Source: CAD feature listing. Evaluate the final solid. Frame: model axes, mm. A direction names the side the tool comes from. Give positions to 0.01 mm unless a question says otherwise; leave off trailing zeros. Write each loop counter-clockwise with the first axis right and the second up, starting at its lowest first coordinate (ties: lowest second). Pieces come first, ordered by that corner, then holes. Notation, with made-up numbers: M -15,80 L -5,80 A10 ccw -5,86 Z; hole C 82.25,12.25 d1. An arc over 180 degrees is marked long. Return JSON: item names as keys, results as strings.
```python
from build123d import *

# Parameters (mm, degrees)
SKETCH2_W               = 200
SKETCH2_H               = 200
BOSS_EXTRUDE1_DEPTH     = 50
CUT_EXTRUDE1_DEPTH      = 151
CUT_EXTRUDE1_DEPTH_BACK = 15
SKETCH5_R               = 75.5
CUT_EXTRUDE2_DEPTH      = 146.688022843
CUT_EXTRUDE2_DEPTH_BACK = 146.688022843
SKETCH7_R               = 50.25
SKETCH12_R              = 20.123320675
BOSS_EXTRUDE2_DEPTH     = 50
CIRPATTERN1_COUNT       = 4
CIRPATTERN1_ANGLE       = 276
SKETCH13_R              = 1.5
CUT_EXTRUDE3_DEPTH      = 10
CIRPATTERN2_COUNT       = 6
BOSS_EXTRUDE3_START     = -8
SKETCH14_R              = 50.25
BOSS_EXTRUDE3_DEPTH     = 8


with BuildPart() as part:
    # Sketch2 → Boss-Extrude1 (new body)
    with BuildSketch(Plane(origin=(0, 0, 0), x_dir=(1, 0, 0), z_dir=(0, 1, 0))):
        Rectangle(SKETCH2_W, SKETCH2_H)
    extrude(amount=BOSS_EXTRUDE1_DEPTH)

    # Sketch5 → Cut-Extrude1 (cut, two sides: drawn at the far end of the back side and taken through both)
    with BuildSketch(Plane(origin=(0, 50, 0), x_dir=(1, 0, 0), z_dir=(0, 1, 0)).offset(-CUT_EXTRUDE1_DEPTH_BACK)):
        with Locations(Location((0, 0, 0), (0, 0, 90))):
            Circle(SKETCH5_R)
    extrude(amount=CUT_EXTRUDE1_DEPTH + CUT_EXTRUDE1_DEPTH_BACK, mode=Mode.SUBTRACT)

    # Sketch7 → Cut-Extrude2 (cut, two sides: drawn at the far end of the back side and taken through both)
    with BuildSketch(Plane(origin=(0, 35, 0), x_dir=(1, 0, 0), z_dir=(0, 1, 0)).offset(-CUT_EXTRUDE2_DEPTH_BACK)):
        with Locations(Location((0, 0, 0), (0, 0, 270))):
            Circle(SKETCH7_R)
    extrude(amount=CUT_EXTRUDE2_DEPTH + CUT_EXTRUDE2_DEPTH_BACK, mode=Mode.SUBTRACT)

    # Sketch12 → Boss-Extrude2 (add)
    with BuildSketch(Plane.XZ):
        with Locations(Location((-74.168810486, 63.963412144, 0), (0, 0, 270))):
            Circle(SKETCH12_R)
    boss_extrude2 = extrude(amount=BOSS_EXTRUDE2_DEPTH)

    # CirPattern1: Boss-Extrude2 ×4 about axis
    cirpattern1_axis = Axis((0, 0, 0), (0, 1, 0))
    for i in range(1, CIRPATTERN1_COUNT):
        add(boss_extrude2.rotate(cirpattern1_axis, i * CIRPATTERN1_ANGLE / (CIRPATTERN1_COUNT - 1)))

    # Sketch13 → Cut-Extrude3 (cut)
    with BuildSketch(Plane(origin=(0, 35, 0), x_dir=(1, 0, 0), z_dir=(0, 1, 0))):
        with Locations(Location((0, 65, 0), (0, 0, 270))):
            Circle(SKETCH13_R)
    cut_extrude3 = extrude(amount=-CUT_EXTRUDE3_DEPTH, mode=Mode.SUBTRACT)

    # CirPattern2: Cut-Extrude3 ×6 about axis
    cirpattern2_axis = Axis((0, 0, 0), (0, 1, 0))
    for i in range(1, CIRPATTERN2_COUNT):
        add(cut_extrude3.rotate(cirpattern2_axis, i * 360 / CIRPATTERN2_COUNT), mode=Mode.SUBTRACT)

    # Sketch14 → Boss-Extrude3 (add)
    with BuildSketch(Plane.XZ.offset(BOSS_EXTRUDE3_START)):
        with Locations(Location((0, 0, 0), (0, 0, 90))):
            Circle(SKETCH14_R)
    extrude(amount=BOSS_EXTRUDE3_DEPTH)


solid = part.part
```
1) Cut plane B-B, the plane y = 11.5. Return the cut outline in (x, z), then the cut area to 3 significant figures.
Numbers:
{"outline": "M -100,-100 L 100,-100 L 100,100 L -100,100 Z; hole C 0,0 d100.5", "area": "32,100 mm²"}
2) Cut plane D-D, the plane y = -33.5. Return the cut outline in (x, z).
Numbers:
{"outline": "C -74.17,63.96 d40.25; C -71.37,-67.08 d40.25; C 66.51,71.89 d40.25; C 69.53,-68.98 d40.25"}
3) Draft query along X for faces 1 (the face through (100, 25, 1)), 2 (the face through (-1, 0, -1)), 3 (the face through (49, 35, -16)), 4 (the face through (-74, -50, 64)). Return one class per face: released by +X, released by -X, zero draft, split by the parting line, or undercut.
Numbers:
{"face 1": "released by +X", "face 2": "undercut", "face 3": "undercut", "face 4": "zero draft"}
4) Cut plane A-A, the plane z = 0. Return the cut outline in (x, y), then the cut area to 3 significant figures.
Numbers:
{"outline": "M -100,0 L 100,0 L 100,50 L 75.5,50 L 75.5,35 L 50.25,35 L 50.25,8 L -50.25,8 L -50.25,35 L -75.5,35 L -75.5,50 L -100,50 Z", "area": "5,020 mm²"}
5) Cut plane C-C, the plane x = -14. Return the cut outline in (y, z), then the cut area to 3 significant figures.
Numbers:
{"outline": "M 0,-100 L 50,-100 L 50,-74.19 L 35,-74.19 L 35,-48.26 L 8,-48.26 L 8,48.26 L 35,48.26 L 35,74.19 L 50,74.19 L 50,100 L 0,100 Z", "area": "5,170 mm²"}
6) Contact query for flat-ended pins moving along their axis: pin 1 Ø8 at (x, z) = (68, 30.5) entering from +Y; pin 2 Ø2.5 at (x, z) = (56.5, 32.5) entering from +Y; pin 3 Ø4 at (x, z) = (58.5, 9) entering from -Y; pin 4 Ø8 at (y, z) = (-27.5, 64) entering from -X. Output: stop coordinate, or through.
Numbers:
{"pin 1": "stops at y = 50", "pin 2": "stops at y = 25", "pin 3": "stops at y = 0", "pin 4": "stops at x = -94.29"}
7) Line query: line 1 (X direction, y = 23, z = 0); line 2 (X direction, y = 27.75, z = -32.5). Output: solid intervals per line, ascending. Write a range as [from, to].
Numbers:
{"line 1": "x = [-100, -50.25], [50.25, 100]", "line 2": "x = [-100, -57.79], [-54.79, -38.33], [38.33, 54.79], [57.79, 100]"}
8) Set-up query: faces 5 (the face through (-1, 8, -1)), 6 (the face through (-68, 50, -46)), 7 (the face through (49.44, -24.65, -70.2)). Return all of +Z, -Z, +X, -X, +Y, -Y with unobstructed straight access to the full face (end or side cutting, diameter ignored); none if empty.
Numbers:
{"face 5": "+Y", "face 6": "+Z, -Z, +X, -X, +Y", "face 7": "-Y"}
